from build123d import *
from OCP.BRepFilletAPI import BRepFilletAPI_MakeChamfer

# Parameters (mm, degrees)
SKETCH1_R           = 9
BOSS_EXTRUDE1_DEPTH = 6.75
CHAMFER1_SIZE       = 6.75
CHAMFER1_SIZE_2     = 1.19020712


with BuildPart() as part:
    # Sketch1 → Boss-Extrude1 (new body)
    with BuildSketch(Plane(origin=(0, 0, 0), x_dir=(1, 0, 0), z_dir=(0, 1, 0))):
        Polygon((-45.420560748, -63.588785047), (-18.420560748, -63.588785047), (62.579439252, -63.588785047), (62.579439252, 98.411214953), (-45.420560748, 98.411214953), (-45.420560748, -36.588785047), align=None)
        with Locations(Location((-18.420560748, -36.588785047, 0), (0, 0, 270))):
            Circle(SKETCH1_R, mode=Mode.SUBTRACT)
        with Locations(Location((35.579439252, 71.411214953, 0), (0, 0, 90))):
            Circle(SKETCH1_R, mode=Mode.SUBTRACT)
        with Locations(Location((35.579439252, 17.411214953, 0), (0, 0, 90))):
            Circle(SKETCH1_R, mode=Mode.SUBTRACT)
        with Locations(Location((-18.420560748, 17.411214953, 0), (0, 0, 270))):
            Circle(SKETCH1_R, mode=Mode.SUBTRACT)
        with Locations(Location((-18.420560748, 71.411214953, 0), (0, 0, 270))):
            Circle(SKETCH1_R, mode=Mode.SUBTRACT)
        with Locations(Location((35.579439252, -36.588785047, 0), (0, 0, 90))):
            Circle(SKETCH1_R, mode=Mode.SUBTRACT)
    extrude(amount=BOSS_EXTRUDE1_DEPTH)

    # Chamfer1
    chamfer1_edges_1 = [part.edges().sort_by_distance(p)[0] for p in [
        (62.579439252, 6.75, -17.411214953),
    ]]
    chamfer1_side_1 = [part.faces().sort_by_distance(p)[0] for p in [
        (62.579439252, 6.726195858, -17.411214953),
    ]]
    chamfer1_edges_2 = [part.edges().sort_by_distance(p)[0] for p in [
        (-45.420560748, 6.75, -17.411214953),
    ]]
    chamfer1_side_2 = [part.faces().sort_by_distance(p)[0] for p in [
        (-45.396756605, 6.75, -17.411214953),
    ]]
    chamfer1 = BRepFilletAPI_MakeChamfer(part.part.solid().wrapped)
    for e in chamfer1_edges_1:
        chamfer1.Add(CHAMFER1_SIZE - 0.0001, CHAMFER1_SIZE_2 - 0.0001, e.wrapped, chamfer1_side_1[0].wrapped)
    for e in chamfer1_edges_2:
        chamfer1.Add(CHAMFER1_SIZE_2 - 0.0001, CHAMFER1_SIZE - 0.0001, e.wrapped, chamfer1_side_2[0].wrapped)
    add(Compound.cast(chamfer1.Shape()), mode=Mode.REPLACE)  # a hair under: the kernel refuses the full size


solid = part.part
Verification items for the finished model (mm, model axes). Give positions to 0.01 mm unless a question says otherwise; leave off trailing zeros. Loops run counter-clockwise (first coordinate to the right, second up) from the corner with the lowest first, then second, coordinate; pieces in that order, holes last.
1) Sectioned sample at C-C, the plane y = 2.75. Enter the section's corners in (x, z), then the cut area to 3 significant figures.
2) Sectioned sample at A-A, the plane x = 43. Enter the section's corners in (y, z), then the cut area to 3 significant figures.
3) Sectioned sample at B-B, the plane z = -12. Count the separate pieces of the cut face and the enclosed holes in it, then the cut area to 3 significant figures.
4) Depth check by flat-ended pin: pin 1 Ø2 at (y, z) = (6, 35) entering from -X; pin 2 Ø16 at (x, z) = (-18.42, -17.41) entering from +Y (3 decimals); pin 3 Ø2 at (y, z) = (5, -82) entering from -X. Enter the tip coordinate at first touch or a pass-through.
5) Thickness scan on line 1 along Z through (x, y) = (-14.5, 5.25); line 2 along X through (y, z) = (6, -76); line 3 along Z through (x, y) = (31, 5.75). Record the ranges inside material, lowest first.
6) Sectioned sample at D-D, the plane x = 30. Enter the section's corners in (y, z), then the cut area to 3 significant figures.
7) Draft check along Z on faces 1 (the flat face through (9, 3, -98.411)), 2 (the flat face through (61.976, 3.422, -16.277)), 3 (the flat face through (8, 3, 63.589)), 4 (the cylindrical face through (-23.9, 3.33, -24.55)). Enter one of: pulls with the +Z half, pulls with the -Z half, needs draft (parallel to the pull), parting line crosses it, or undercut.
Answers:
1. outline: (-44.94, -98.41) - (62.09, -98.41) - (62.09, 63.59) - (-44.94, 63.59) - close; hole circle Ø18 at (-18.42, -71.41); hole circle Ø18 at (-18.42, -17.41); hole circle Ø18 at (-18.42, 36.59); hole circle Ø18 at (35.58, -71.41); hole circle Ø18 at (35.58, -17.41); hole circle Ø18 at (35.58, 36.59)
1. area: 15,800 mm2
2. outline: (0, -98.41) - (6.75, -98.41) - (6.75, -76.5) - (0, -76.5) - close; (0, -66.32) - (6.75, -66.32) - (6.75, -22.5) - (0, -22.5) - close; (0, -12.32) - (6.75, -12.32) - (6.75, 31.5) - (0, 31.5) - close; (0, 41.68) - (6.75, 41.68) - (6.75, 63.59) - (0, 63.59) - close
2. area: 887 mm2
3. separate pieces: 3
3. enclosed holes: 0
3. area: 527 mm2
4. pin 1: stops at x = -44.54
4. pin 2: passes through
4. pin 3: stops at x = -44.72
5. line 1: z = -98.41 to -79.51, -63.31 to -25.51, -9.31 to 28.49, 44.69 to 63.59
5. line 2: x = -44.36 to -26.16, -10.68 to 27.84, 43.32 to 61.52
5. line 3: z = -98.41 to -79.16, -63.66 to -25.16, -9.66 to 28.84, 44.34 to 63.59
6. outline: (0, -98.41) - (6.75, -98.41) - (6.75, -78.47) - (0, -78.47) - close; (0, -64.35) - (6.75, -64.35) - (6.75, -24.47) - (0, -24.47) - close; (0, -10.35) - (6.75, -10.35) - (6.75, 29.53) - (0, 29.53) - close; (0, 43.65) - (6.75, 43.65) - (6.75, 63.59) - (0, 63.59) - close
6. area: 807 mm2
7. face 1: pulls with the -Z half
7. face 2: needs draft
7. face 3: pulls with the +Z half
7. face 4: undercut
